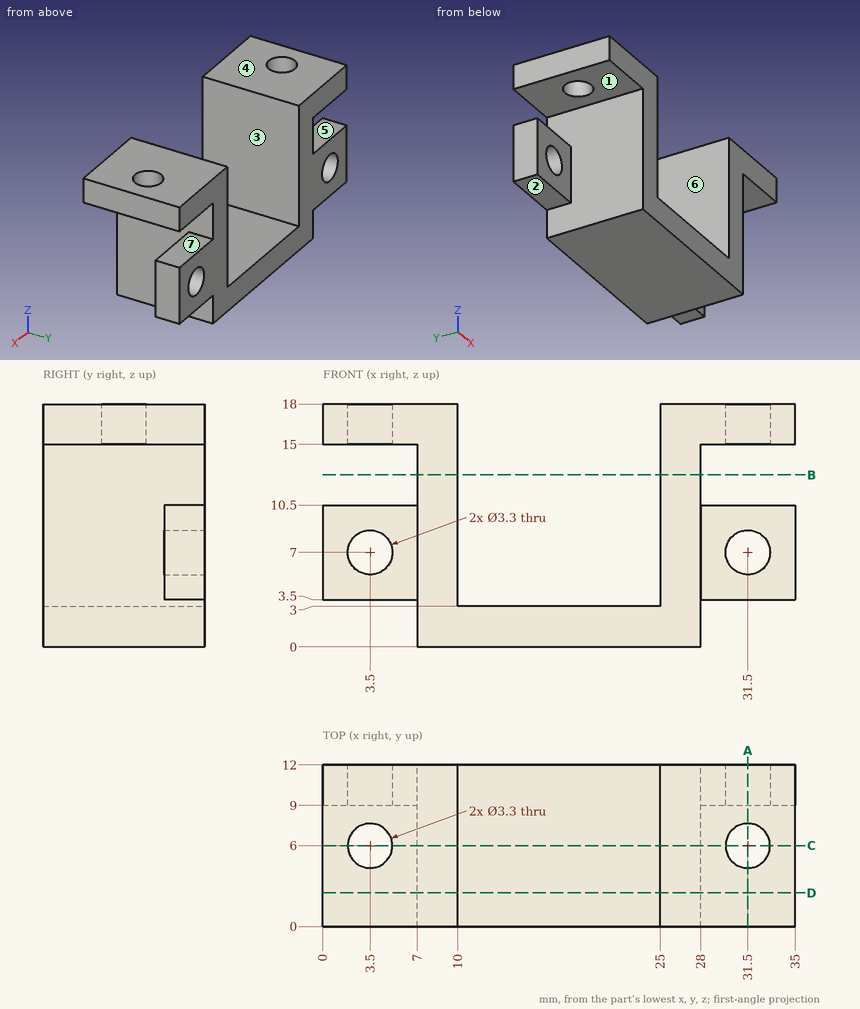
Check sheet for the drawn part. Datum: minimum x, y, z corner. Units: mm. A direction names the side the tool comes from. Give positions to 0.01 mm unless a question says otherwise; leave off trailing zeros. Write each loop counter-clockwise with the first axis right and the second up, starting at its lowest first coordinate (ties: lowest second). Pieces come first, ordered by that corner, then holes.
(1) Access from +Z, -Z, +X, -X, +Y, -Y to the whole of each face (thin tool, end or side, straight path). Record for the marked faces 1, 2 and 3.
(2) Mould release check, pull along Z, two halves, no side actions. Record for the marked faces 4, 5, 6 and 7: +Z half, -Z half, draft (parallel to the pull), parting line (faces both ways), or undercut.
(3) Material ranges on line 1 (X direction, y = 11.2, z = 7); line 2 (Z direction, x = 31.5, y = 9.65); line 3 (X direction, y = 4.75, z = 6.5), recorded low to high.
(4) Cross-section at B-B (z = 12.75). Enter the section's corners in (x, y), plus the area to 3 significant figures.
(5) Cross-section at A-A (x = 31.5). Enter the section's corners in (y, z), plus the area to 3 significant figures.
(6) Gauge pin test, flat ends, axial feed: pin 1 (1 mm diameter, centred on x = 31, z = 11.5, fed in from +Y); pin 2 (2 mm diameter, centred on x = 2.5, z = 6.5, fed in from -Y); pin 3 (6 mm diameter, centred on x = 20, y = 7, fed in from +Z); pin 4 (3.5 mm diameter, centred on x = 2.5, y = 11, fed in from -Z). Record the tip position at first contact, or that the pin passes through.
(7) Cross-section at C-C (y = 6). Enter the section's corners in (x, z).
(8) Cross-section at D-D (y = 2.5). Enter the section's corners in (x, z), plus the area to 3 significant figures.
Worked out:
1. face 1: -X, +Y, -Y
1. face 2: -Z, -X, +Y, -Y
1. face 3: +Z, +Y, -Y
2. face 4: +Z half
2. face 5: undercut
2. face 6: draft
2. face 7: undercut
3. line 1: x = 0 to 1.85, 5.15 to 10, 25 to 29.85, 33.15 to 35
3. line 2: z = 3.5 to 5.35, 8.65 to 10.5, 15 to 18
3. line 3: x = 7 to 10, 25 to 28
4. outline: (7, 0) - (10, 0) - (10, 12) - (7, 12) - close; (25, 0) - (28, 0) - (28, 12) - (25, 12) - close
4. area: 72.0 mm2
5. outline: (0, 15) - (4.35, 15) - (4.35, 18) - (0, 18) - close; (7.65, 15) - (12, 15) - (12, 18) - (7.65, 18) - close; (9, 3.5) - (12, 3.5) - (12, 5.35) - (9, 5.35) - close; (9, 8.65) - (12, 8.65) - (12, 10.5) - (9, 10.5) - close
5. area: 37.2 mm2
6. pin 1: passes through
6. pin 2: stops at y = 9
6. pin 3: stops at z = 3
6. pin 4: stops at z = 3.5
7. outline: (0, 15) - (1.85, 15) - (1.85, 18) - (0, 18) - close; (5.15, 15) - (7, 15) - (7, 0) - (28, 0) - (28, 15) - (29.85, 15) - (29.85, 18) - (25, 18) - (25, 3) - (10, 3) - (10, 18) - (5.15, 18) - close; (33.15, 15) - (35, 15) - (35, 18) - (33.15, 18) - close
8. outline: (0, 15) - (7, 15) - (7, 0) - (28, 0) - (28, 15) - (35, 15) - (35, 18) - (25, 18) - (25, 3) - (10, 3) - (10, 18) - (0, 18) - close
8. area: 195 mm2
